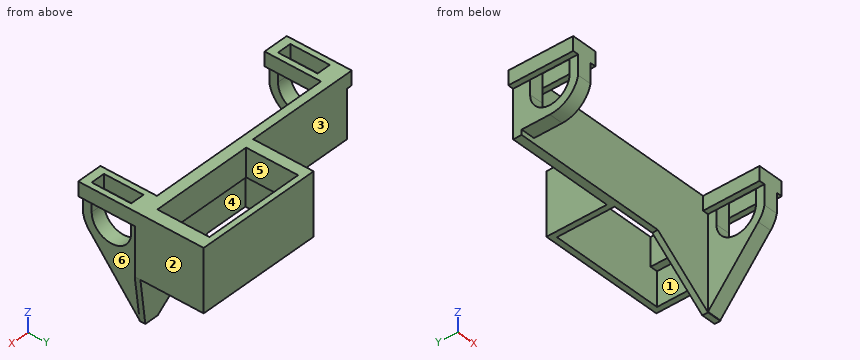
```python
from build123d import *

# Parameters (mm, degrees)
SKETCH014_W   = 40.6
SKETCH014_H   = 20.4
PAD013_DEPTH  = 22
PAD014_DEPTH  = 2
PAD012_DEPTH  = 5
SKETCH016_W   = 9
SKETCH016_H   = 22
SKETCH016_W_2 = 5
SKETCH016_H_2 = 17
PAD015_DEPTH  = 5
SKETCH017_W   = 44.6
SKETCH017_H   = 24.4
SKETCH017_W_2 = 36
SKETCH017_H_2 = 18.4
PAD016_DEPTH  = 10
PAD017_DEPTH  = 5
SKETCH019_W   = 9
SKETCH019_H   = 23
SKETCH019_W_2 = 5
SKETCH019_H_2 = 17
PAD018_DEPTH  = 5


with BuildPart() as part:
    # Sketch014 → Pad013 (new body)
    with BuildSketch(Plane.XY):
        Polygon((-2, 22.4), (42.6, 22.4), (42.6, -2), (-40, -2), (-40, 1), (-2, 1), align=None)
        with Locations((20.3, 10.2)):
            Rectangle(SKETCH014_W, SKETCH014_H, mode=Mode.SUBTRACT)
    extrude(amount=PAD013_DEPTH)

    # Sketch015 → Pad014 (join)
    with BuildSketch(Plane.XZ):
        Polygon((0, 12), (35.6, -16), (40.6, -16), (42.6, 0), (42.6, 12), align=None)
    extrude(amount=PAD014_DEPTH)

    # Sketch013 → Pad012 (join)
    with BuildSketch(Plane(origin=(40.6, 0, 10), x_dir=(0, 1, 0), z_dir=(1, 0, 0))):
        with BuildLine():
            Line((-22, 12), (-22, 0))
            ThreePointArc((-22, 0), (-21.192692, -2.415248), (-19.812151, -4.555173))
            Line((-19.812151, -4.555173), (-2, -25.782868))
            Line((-2, -25.782868), (-2, 2))
            Line((-2, 12), (-2, 2))
            Line((-5, 12), (-2, 12))
            Line((-5, 2), (-5, 12))
            ThreePointArc((-19, 2), (-12, -5), (-5, 2))
            Line((-19, 12), (-19, 2))
            Line((-22, 12), (-19, 12))
        make_face()
    extrude(amount=-PAD012_DEPTH)

    # Sketch016 → Pad015 (join)
    with BuildSketch(Plane(origin=(35.6, 0, 22), x_dir=(1, 0, 0), z_dir=(0, 0, 1))):
        with Locations((2.5, -11)):
            Rectangle(SKETCH016_W, SKETCH016_H)
        with Locations((2.5, -10.5)):
            Rectangle(SKETCH016_W_2, SKETCH016_H_2, mode=Mode.SUBTRACT)
    extrude(amount=-PAD015_DEPTH)

    # Sketch017 → Pad016 (join)
    with BuildSketch(Plane.XY.offset(12)):
        with Locations((20.3, 10.2)):
            Rectangle(SKETCH017_W, SKETCH017_H)
        with Locations((20, 11.2)):
            Rectangle(SKETCH017_W_2, SKETCH017_H_2, mode=Mode.SUBTRACT)
    extrude(amount=PAD016_DEPTH)

    # Sketch018 → Pad017 (join)
    with BuildSketch(Plane(origin=(-40, 0, 10), x_dir=(0, 1, 0), z_dir=(1, 0, 0))):
        with BuildLine():
            Line((-22, 12), (-22, 0))
            ThreePointArc((-22, 0), (-18.465444, -5.886573), (-12, -8.198039))
            Line((-12, -8.198039), (-2, -8.198039))
            Line((-2, -8.198039), (-2, 2))
            Line((-2, 12), (-2, 2))
            Line((-5, 12), (-2, 12))
            Line((-5, 2), (-5, 12))
            ThreePointArc((-19, 2), (-12, -5), (-5, 2))
            Line((-19, 12), (-19, 2))
            Line((-22, 12), (-19, 12))
        make_face()
    extrude(amount=PAD017_DEPTH)

    # Sketch019 → Pad018 (join)
    with BuildSketch(Plane(origin=(-40, 0, 22), x_dir=(1, 0, 0), z_dir=(0, 0, 1))):
        with Locations((2.5, -10.5)):
            Rectangle(SKETCH019_W, SKETCH019_H)
        with Locations((2.5, -10.5)):
            Rectangle(SKETCH019_W_2, SKETCH019_H_2, mode=Mode.SUBTRACT)
    extrude(amount=-PAD018_DEPTH)


solid = part.part
```
For this review, take the finished solid that the model builds, in its own axes (mm). Face numbers are marked on the shaded views. A direction names the side the tool comes from. Round coordinates to 2 decimals unless told otherwise and drop trailing zeros. Write each loop counter-clockwise with the first axis right and the second up, starting at its lowest first coordinate (ties: lowest second). Pieces come first, ordered by that corner, then holes. Notation, with made-up numbers: M 21,83.5 L 65,83.5 A22 ccw 65,96.5 Z; hole C 28,86.25 d6. An arc over 180 degrees is marked long. One line per item, written item: value. Start each with the question number.
(1) We need section B-B (z = 8). Give the boundary of the cut face in (x, y), and give its area (3 significant figures).
(2) We need section D-D (y = -10). Give the boundary of the cut face in (x, z), and give its area (3 significant figures).
(3) The part is to be moulded in two halves that separate along X. For the marked faces 1, 2 and 3, say which applies: released by +X, released by -X, zero draft, split by the parting line, or undercut.
(4) Insertion check: pin 1 (13.5 mm diameter, centred on y = -15.5, z = 10, fed in from -X); pin 2 (0.6 mm diameter, centred on x = -34, y = -9.5, fed in from -Z); pin 3 (5.5 mm diameter, centred on x = -37, y = -9, fed in from -Z). Each pin has a flat end and moves straight along its axis. Give the tip position at first contact, or say it passes through.
(5) Wall thickness on line 1 (X direction, y = 17, z = 5); line 2 (Y direction, x = 8, z = 8.5); line 3 (X direction, y = 14, z = 17): over which ranges is each line inside the solid? List them lowest first.
(6) We need section A-A (y = 4). Give the boundary of the cut face in (x, z).
(7) Machinability: for the marked faces 4, 5 and 6, which of the approach directions +Z, -Z, +X, -X, +Y, -Y give a long, thin tool a straight path to every point of the face, cutting with its end or side? Answer none if there is none.
(8) We need section C-C (x = 17.5). Give the boundary of the cut face in (y, z).
Result:
1. outline: M -40,-21.38 L -35,-21.38 L -35,-17.74 L -40,-17.74 Z; M -40,-6.26 L -35,-6.26 L -35,-2 L 35.6,-2 L 35.6,-6.26 L 40.6,-6.26 L 40.6,-2 L 42.6,-2 L 42.6,22.4 L -2,22.4 L -2,1 L -40,1 Z; M 35.6,-21.38 L 40.6,-21.38 L 40.6,-17.74 L 35.6,-17.74 Z; hole M 0,0 L 40.6,0 L 40.6,20.4 L 0,20.4 Z
1. area: 453 mm²
2. outline: M -42,17 L -40,17 L -40,22 L -42,22 Z; M -40,1.8 L -35,1.8 L -35,5.29 L -40,5.29 Z; M -35,17 L -33,17 L -33,22 L -35,22 Z; M 33.6,17 L 35.6,17 L 35.6,22 L 33.6,22 Z; M 35.6,-6.25 L 40.6,-6.25 L 40.6,5.29 L 35.6,5.29 Z; M 40.6,17 L 42.6,17 L 42.6,22 L 40.6,22 Z
2. area: 115 mm²
3. face 1: undercut
3. face 2: released by +X
3. face 3: zero draft
4. pin 1: x = -40
4. pin 2: z = 17
4. pin 3: z = 1.8
5. line 1: -2 to 0, 40.6 to 42.6
5. line 2: -2 to 0, 20.4 to 22.4
5. line 3: -2 to 2, 38 to 42.6
6. outline: M -2,0 L 0,0 L 0,12 L 2,12 L 2,22 L -2,22 Z; M 38,12 L 40.6,12 L 40.6,0 L 42.6,0 L 42.6,22 L 38,22 Z
7. face 4: -Z
7. face 5: +Z, -Z
7. face 6: -Z, +X, -Y
8. outline: M -2,-1.76 L 0,-1.76 L 0,12 L 2,12 L 2,22 L -2,22 Z; M 20.4,0 L 22.4,0 L 22.4,22 L 20.4,22 Z
